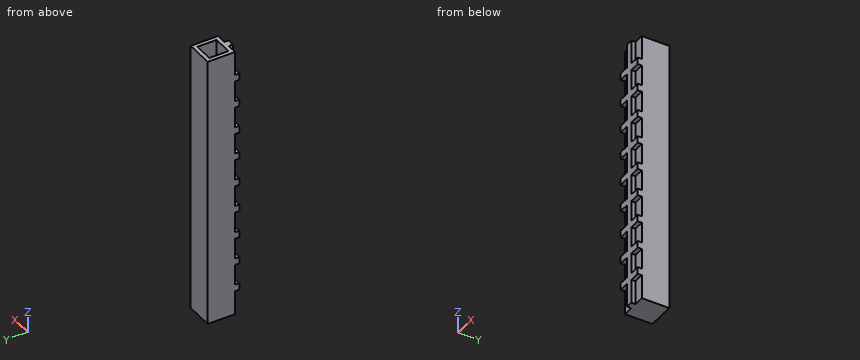
```python
from build123d import *

# Parameters (mm, degrees)
F0_W     = 10
F0_H     = 10
F1_DEPTH = 100
F2_T     = -1.5
F4_DEPTH = 1.5


with BuildPart() as f1:
    # F0 (on Top) → F1 (new body)
    with BuildSketch(Plane.XY):
        Rectangle(F0_W, F0_H)
    extrude(amount=F1_DEPTH)

    # F2
    f2_openings = [f1.faces().sort_by_distance(p)[0] for p in [
        (0, 0, 100),
    ]]
    offset(amount=F2_T, openings=f2_openings)

    # F3 (on face) → F4 (join)
    with BuildSketch(Plane.XZ.offset(5)):
        Polygon((1.25, 100), (-1.25, 100), (-1.25, 91.25), (-5, 91.25), (-5, 88.75), (-1.25, 88.75), (-1.25, 81.25), (-5, 81.25), (-5, 78.75), (-1.25, 78.75), (-1.25, 71.25), (-5, 71.25), (-5, 68.75), (-1.25, 68.75), (-1.25, 61.25), (-5, 61.25), (-5, 58.75), (-1.25, 58.75), (-1.25, 51.25), (-5, 51.25), (-5, 48.75), (-1.25, 48.75), (-1.25, 41.25), (-5, 41.25), (-5, 38.75), (-1.25, 38.75), (-1.25, 31.25), (-5, 31.25), (-5, 28.75), (-1.25, 28.75), (-1.25, 21.25), (-5, 21.25), (-5, 18.75), (-1.25, 18.75), (-1.25, 11.25), (-5, 11.25), (-5, 8.75), (-1.25, 8.75), (-1.25, 0), (1.25, 0), (1.25, 8.75), (5, 8.75), (5, 11.25), (1.25, 11.25), (1.25, 18.75), (5, 18.75), (5, 21.25), (1.25, 21.25), (1.25, 28.75), (5, 28.75), (5, 31.25), (1.25, 31.25), (1.25, 38.75), (5, 38.75), (5, 41.25), (1.25, 41.25), (1.25, 48.75), (5, 48.75), (5, 51.25), (1.25, 51.25), (1.25, 58.75), (5, 58.75), (5, 61.25), (1.25, 61.25), (1.25, 68.75), (5, 68.75), (5, 71.25), (1.25, 71.25), (1.25, 78.75), (5, 78.75), (5, 81.25), (1.25, 81.25), (1.25, 88.75), (5, 88.75), (5, 91.25), (1.25, 91.25), align=None)
    extrude(amount=F4_DEPTH)


solid = f1.part
```
Verification items for the finished model (mm, model axes). Give positions to 0.01 mm unless a question says otherwise; leave off trailing zeros. Write each loop counter-clockwise with the first axis right and the second up, starting at its lowest first coordinate (ties: lowest second). Pieces come first, ordered by that corner, then holes. Notation, with made-up numbers: (1.25, 58) - (53.25, 58) arc R20 cw to (53.25, 68) - close; hole circle Ø9 at (-34.5, 18.5). An arc over 180 degrees is marked (long way). Put each result on its own line as item: value.
Q1. Scan lines: probe 1 along X at (y, z) = (2.75, 8); probe 2 along Y at (x, z) = (3, 79.5). Record each from-to range of solid material in increasing order. Write a range as from..to.
Result:
probe 1: -5..-3.5, 3.5..5
probe 2: -6.5..-3.5, 3.5..5
Q2. Section check B-B on y = 0. Record the cut outline in (x, z).
Result:
outline: (-5, 0) - (5, 0) - (5, 100) - (3.5, 100) - (3.5, 1.5) - (-3.5, 1.5) - (-3.5, 100) - (-5, 100) - close
Q3. Section check C-C on x = 0. Record the cut outline in (y, z).
Result:
outline: (-6.5, 0) - (5, 0) - (5, 100) - (3.5, 100) - (3.5, 1.5) - (-3.5, 1.5) - (-3.5, 100) - (-6.5, 100) - close
Q4. Section check A-A on z = 92.5. Record the cut outline in (x, y).
Result:
outline: (-5, -5) - (-1.25, -5) - (-1.25, -6.5) - (1.25, -6.5) - (1.25, -5) - (5, -5) - (5, 5) - (-5, 5) - close; hole (-3.5, -3.5) - (3.5, -3.5) - (3.5, 3.5) - (-3.5, 3.5) - close
Q5. Depth check by flat-ended pin: P1, Ø4, axis at x = 3.5, z = 25.5, coming from the -Y side; P2, Ø1.2, axis at x = 2.5, y = -6, coming from the -Z side; P3, Ø0.8, axis at y = -5.5, z = 84, coming from the -X side. Enter the tip coordinate at first touch or a pass-through.
Result:
P1: y = -5
P2: z = 8.75
P3: x = -1.25
